Input: part model. Units: mm. Frame: model coordinates. Coordinates: 2 decimals unless noted, no trailing zeros. Order: outer loops, then holes, each group sorted by start corner. A loop starts at its lowest first (then second) coordinate and runs counter-clockwise, first axis right, second up. Notation, with made-up numbers: M 10,16.25 L 22,16.25 A26 cw 22,36.25 Z; hole C 62.5,14.25 d7. An arc over 180 degrees is marked long. One line per item, written item: value.
```python
from build123d import *

# Parameters (mm, degrees)
CROQUIS1_W              = 54.203553954
CROQUIS1_H              = 8.324117214
CROQUIS1_W_2            = 10.370081464
CROQUIS1_H_2            = 27.461512026
CROQUIS1_W_3            = 8.449696009
CROQUIS1_H_3            = 27.269473481
CROQUIS1_W_4            = 18.435700381
CROQUIS1_H_4            = 17.859584744
SALIENTE_EXTRUIR1_DEPTH = 5
CROQUIS3_W              = 111
CROQUIS3_H              = 5
SALIENTE_EXTRUIR2_DEPTH = 6


with BuildPart() as part:
    # Croquis1 → Saliente-Extruir1 (new body)
    with BuildSketch(Plane.XY):
        Polygon((0.553582562, 91.831917191), (0.553582562, 5.331917191), (111.553582562, 5.331917191), (111.553582562, 28.831917191), (87.909456329, 28.831917191), (87.909456329, 86.831917191), (111.553582562, 86.831917191), (111.553582562, 91.831917191), align=None)
        with Locations((56.991342937, 82.669858584)):
            Rectangle(CROQUIS1_W, CROQUIS1_H, mode=Mode.SUBTRACT)
        with Locations((29.145661363, 57.958361113)):
            Rectangle(CROQUIS1_W_2, CROQUIS1_H_2, mode=Mode.SUBTRACT)
        with Locations((70.625987221, 41.966653932)):
            Rectangle(CROQUIS1_W_3, CROQUIS1_H_3, mode=Mode.SUBTRACT)
        with Locations((54.686787933, 60.902124819)):
            Rectangle(CROQUIS1_W_4, CROQUIS1_H_4, mode=Mode.SUBTRACT)
    extrude(amount=SALIENTE_EXTRUIR1_DEPTH)

    # Croquis3 → Saliente-Extruir2 (add)
    with BuildSketch(Plane.XZ.offset(-5.331917191)):
        with Locations((56.053582562, 2.5)):
            Rectangle(CROQUIS3_W, CROQUIS3_H)
    extrude(amount=SALIENTE_EXTRUIR2_DEPTH)


solid = part.part
```
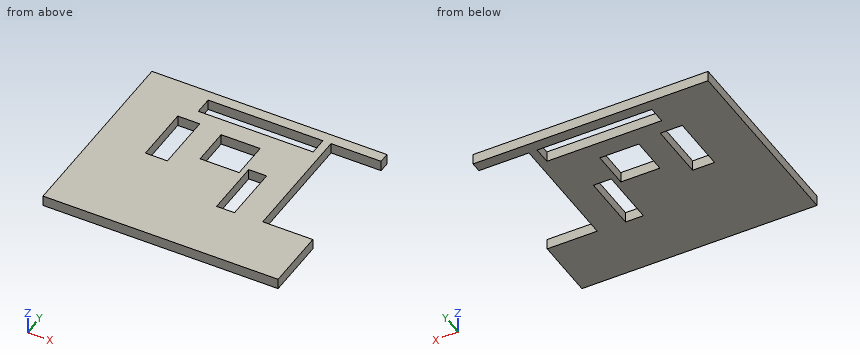
(1) Cut plane A-A on x = 38.5. Output: boundary loops of the cut face in (y, z), plus the area to 3 significant figures.
Data:
outline: M -0.67,0 L 78.51,0 L 78.51,5 L -0.67,5 Z; M 86.83,0 L 91.83,0 L 91.83,5 L 86.83,5 Z
area: 421 mm2
(2) Cut plane C-C on x = 72. Output: boundary loops of the cut face in (y, z).
Data:
outline: M -0.67,0 L 28.33,0 L 28.33,5 L -0.67,5 Z; M 55.6,0 L 78.51,0 L 78.51,5 L 55.6,5 Z; M 86.83,0 L 91.83,0 L 91.83,5 L 86.83,5 Z
(3) Cut plane B-B on y = 63.5. Output: boundary loops of the cut face in (x, z), plus the area to 3 significant figures.
Data:
outline: M 0.55,0 L 23.96,0 L 23.96,5 L 0.55,5 Z; M 34.33,0 L 45.47,0 L 45.47,5 L 34.33,5 Z; M 63.9,0 L 87.91,0 L 87.91,5 L 63.9,5 Z
area: 293 mm2
(4) Ray query, line 1 (Y direction, x = 71.5, z = 3.8); line 2 (Y direction, x = 59, z = 3.15); line 3 (X direction, y = 44.5, z = 0.7). Return the intervals inside material, ascending. Write a range as from..to.
Data:
line 1: y = -0.67..28.33, 55.6..78.51, 86.83..91.83
line 2: y = -0.67..51.97, 69.83..78.51, 86.83..91.83
line 3: x = 0.55..23.96, 34.33..66.4, 74.85..87.91
(5) First-contact query: pin 1 (2.5 mm diameter, centred on y = 64.5, z = 3.5, fed in from +X). Flat tip, straight axial feed; report the tip coordinate or a pass-through.
Data:
pin 1: stops at x = 87.91
(6) Cut plane D-D on z = 3.65. Output: boundary loops of the cut face in (x, y), plus the area to 3 significant figures.
Data:
outline: M 0.55,-0.67 L 111.55,-0.67 L 111.55,28.83 L 87.91,28.83 L 87.91,86.83 L 111.55,86.83 L 111.55,91.83 L 0.55,91.83 Z; hole M 23.96,44.23 L 34.33,44.23 L 34.33,71.69 L 23.96,71.69 Z; hole M 29.89,78.51 L 84.09,78.51 L 84.09,86.83 L 29.89,86.83 Z; hole M 45.47,51.97 L 63.9,51.97 L 63.9,69.83 L 45.47,69.83 Z; hole M 66.4,28.33 L 74.85,28.33 L 74.85,55.6 L 66.4,55.6 Z
area: 7,600 mm2
